Design review of the part built by this model. Coordinates are the model's own, in mm. Give positions to 0.01 mm unless a question says otherwise; leave off trailing zeros. Order: outer loops, then holes, each group sorted by start corner. A loop starts at its lowest first (then second) coordinate and runs counter-clockwise, first axis right, second up. Notation, with made-up numbers: (59.25, -2) -> (81.25, -2) arc R12 ccw to (81.25, 18) -> close; hole circle Ø7 at (39, 65). An arc over 180 degrees is marked (long way). Return JSON: item names as keys, results as strings.
```python
from build123d import *

# Parameters (mm, degrees)
SKETCH1_R                   = 48.006
BOSS_EXTRUDE1_DEPTH         = 3.175
SKETCH2_R                   = 46.482
BOSS_EXTRUDE2_DEPTH         = 3.175
F_1_4_CLEARANCE_HOLE1_D     = 6.7564
F_1_4_CLEARANCE_HOLE1_DEPTH = 48.770172657
F_1_4_CLEARANCE_HOLE1_TIP   = 2.029827343


with BuildPart() as part:
    # Sketch1 → Boss-Extrude1 (new body)
    with BuildSketch(Plane(origin=(0, 0, 0), x_dir=(1, 0, 0), z_dir=(0, 1, 0))):
        Circle(SKETCH1_R)
    extrude(amount=BOSS_EXTRUDE1_DEPTH)

    # Sketch2 → Boss-Extrude2 (add)
    with BuildSketch(Plane(origin=(0, 3.175, 0), x_dir=(1, 0, 0), z_dir=(0, 1, 0))):
        Circle(SKETCH2_R)
    extrude(amount=BOSS_EXTRUDE2_DEPTH)

    # 1/4 Clearance Hole1
    with Locations(Plane(origin=(0, 0, 0), x_dir=(-1, 0, 0), z_dir=(0, -1, 0))):
        with Locations((-25.4, 0), (0, 0), (25.4, 0)):
            Hole(F_1_4_CLEARANCE_HOLE1_D / 2, depth=F_1_4_CLEARANCE_HOLE1_DEPTH)
            with Locations((0, 0, -(F_1_4_CLEARANCE_HOLE1_DEPTH + F_1_4_CLEARANCE_HOLE1_TIP / 2))):  # 118° drill point
                Cone(0, F_1_4_CLEARANCE_HOLE1_D / 2, F_1_4_CLEARANCE_HOLE1_TIP, mode=Mode.SUBTRACT)


solid = part.part
```
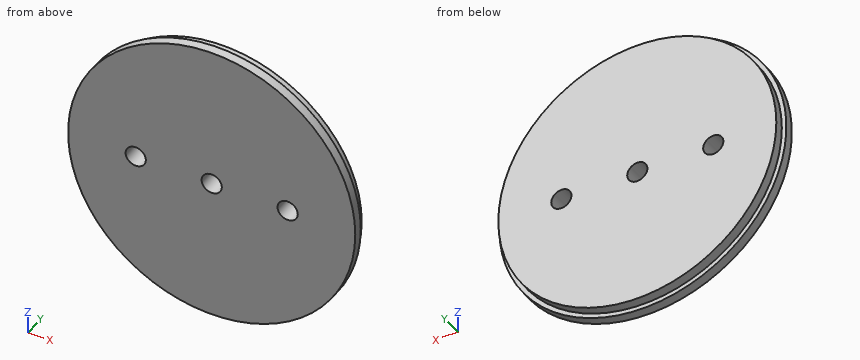
Item 1: Add section D-D (z = -30). Give the boundary of the cut face in (x, y) (3 decimals).
Result set:
{"outline": "(-37.478, 0) -> (37.478, 0) -> (37.478, 3.175) -> (35.505, 3.175) -> (35.505, 6.35) -> (-35.505, 6.35) -> (-35.505, 3.175) -> (-37.478, 3.175) -> close"}
Item 2: Add section C-C (y = 4.5). Give the boundary of the cut face in (x, z).
Result set:
{"outline": "circle Ø92.96 at (0, 0); hole circle Ø6.76 at (-25.4, 0); hole circle Ø6.76 at (0, 0); hole circle Ø6.76 at (25.4, 0)"}
Item 3: Add section B-B (z = 0). Give the boundary of the cut face in (x, y) (3 decimals), plus the area to 3 significant figures.
Result set:
{"outline": "(-48.006, 0) -> (-28.778, 0) -> (-28.778, 6.35) -> (-46.482, 6.35) -> (-46.482, 3.175) -> (-48.006, 3.175) -> close; (-22.022, 0) -> (-3.378, 0) -> (-3.378, 6.35) -> (-22.022, 6.35) -> close; (3.378, 0) -> (22.022, 0) -> (22.022, 6.35) -> (3.378, 6.35) -> close; (28.778, 0) -> (48.006, 0) -> (48.006, 3.175) -> (46.482, 3.175) -> (46.482, 6.35) -> (28.778, 6.35) -> close", "area": "471 mm^2"}
Item 4: Wall thickness on L1, parallel to Z at x = 25.4, y = 2; L2, parallel to Z at x = 28, y = 4; L3, parallel to Y at x = 40, z = 26 (3 decimals): over which ranges is each line inside the solid? List them lowest first. Write a range as [from, to].
Result set:
{"L1": "z = [-40.74, -3.38], [3.38, 40.74]", "L2": "z = [-37.1, -2.16], [2.16, 37.1]", "L3": "y = [0, 3.175]"}
Item 5: Add section A-A (x = 0). Give the boundary of the cut face in (y, z) (3 decimals).
Result set:
{"outline": "(0, -48.006) -> (3.175, -48.006) -> (3.175, -46.482) -> (6.35, -46.482) -> (6.35, -3.378) -> (0, -3.378) -> close; (0, 3.378) -> (6.35, 3.378) -> (6.35, 46.482) -> (3.175, 46.482) -> (3.175, 48.006) -> (0, 48.006) -> close"}
